Autodesk Inventor part; units mm, degrees
ref_plane "YZ Plane" through (0, 0, 0) normal (1, 0, 0) x (0, 1, 0)
ref_plane "XZ Plane" through (0, 0, 0) normal (0, 1, 0) x (-1, 0, 0)
ref_plane "XY Plane" through (0, 0, 0) normal (0, 0, 1) x (1, 0, 0)
sketch "スケッチ1" plane through (0, 0, 0) normal (0, 0, 1) x (1, 0, 0)
  line L0 (-20, -8.9) -> (20, -8.9)
  line L1 (20, -8.9) -> (20, 8.9)
  line L2 (20, 8.9) -> (-20, 8.9)
  line L3 (-20, 8.9) -> (-20, -8.9)
  line L4 (-20, -8.9) -> (20, 8.9) construction
  line L5 (20, -8.9) -> (-20, 8.9) construction
  circle A0 centre (0, 0) radius 2.1
  circle A1 centre (10, 0) radius 2.1
  circle A2 centre (-10, 0) radius 2.1
  dimension "d0" = 40
  dimension "d1" = 17.8
  dimension "d2" = 4.2
  dimension "d3" = 4.2
  dimension "d4" = 4.2
extrude "押し出し1" add sketch "スケッチ1" along normal blind 0.4
chamfer "面取り1" distance 2 distance2 0.2 1 edges at (0, 8.9, 0.4) measured on face at (0.0844, -6.6282, 0.4)
chamfer "面取り2" distance 0.2 distance2 2 1 edges at (0, 8.9, 0) measured on face at (-6.6667, 8.9, 0.0667)
sketch "スケッチ2" plane through (0, 0, 0.4) normal (0, 0, 1) x (1, 0, 0)
  circle A0 centre (-16, 0) radius 1.7
  point P0 (0, 0)
  dimension "d13" = 3.4
extrude "押し出し2" cut sketch "スケッチ2" against normal blind 10
properties part number "cutter_XB210" material "鋼 AISI 1015"
Input: part model. Units: mm. Frame: model coordinates. Give positions to 0.01 mm unless a question says otherwise; leave off trailing zeros. Write each loop counter-clockwise with the first axis right and the second up, starting at its lowest first coordinate (ties: lowest second). Pieces come first, ordered by that corner, then holes. Notation, with made-up numbers: M -31.75,-34.5 L 18.25,-34.5 A30 ccw 18.25,0.5 Z; hole C 7.25,57.25 d9. An arc over 180 degrees is marked long. Use one line per item in the form item = value.
1. Ray query, L1, parallel to X at y = 1.25, z = 0.3. Return the intervals inside material, ascending.
Outcome:
L1 = -20 to -17.15, -14.85 to -11.69, -8.31 to -1.69, 1.69 to 8.31, 11.69 to 20
2. Mould query, pull axis X, two halves, no side actions, for faces 1 (the face through (7.9, -0.09, 0.2)), 2 (the face through (0, -3, 0.4)), 3 (the face through (-12.1, -0.09, 0.2)). Classes: released by +X, released by -X, zero draft, split by the parting line, or undercut.
Outcome:
face_1 = undercut
face_2 = zero draft
face_3 = undercut
3. Cut plane B-B on y = 0. Return loops of the section in (x, z).
Outcome:
outline = M -20,0 L -17.7,0 L -17.7,0.4 L -20,0.4 Z; M -14.3,0 L -12.1,0 L -12.1,0.4 L -14.3,0.4 Z; M -7.9,0 L -2.1,0 L -2.1,0.4 L -7.9,0.4 Z; M 2.1,0 L 7.9,0 L 7.9,0.4 L 2.1,0.4 Z; M 12.1,0 L 20,0 L 20,0.4 L 12.1,0.4 Z
4. First-contact query: P1, Ø4, axis at x = -16, y = 0, coming from the -Z side; P2, Ø4, axis at x = 0, y = 0, coming from the +Z side. Flat tips, straight axial feed; report the tip coordinate or a pass-through.
Outcome:
P1 = 0
P2 = through
5. Cut plane C-C on z = 0.3. Return loops of the section in (x, y), and give its area (3 significant figures).
Outcome:
outline = M -20,-8.9 L 20,-8.9 L 20,7.9 L -20,7.9 Z; hole C -16,0 d3.4; hole C -10,0 d4.2; hole C 0,0 d4.2; hole C 10,0 d4.2
area = 621 mm²
